```python
from build123d import *

# Parameters (mm, degrees)
RESSALTO_EXTRUS_O1_DEPTH = 30
ESBO_O2_R                = 5
CORTE_EXTRUS_O1_DEPTH    = 30
FILETE1_R                = 10


with BuildPart() as part:
    # Esboço1 → Ressalto-extrusão1 (new body)
    with BuildSketch(Plane.XY):
        with BuildLine():
            Line((-51.174680709, 2.345199545), (-29.908193511, 2.345199545))
            ThreePointArc((-29.908193511, 2.345199545), (0, 30), (29.908193511, 2.345199545))
            Line((29.908193511, 2.345199545), (51.174680709, 2.345199545))
            Line((51.174680709, 2.345199545), (78.983139003, 2.345199545))
            Line((78.983139003, 2.345199545), (78.983139003, 15))
            Line((78.983139003, 15), (48.983139003, 15))
            ThreePointArc((48.983139003, 15), (0, 51.228389654), (-48.983139003, 15))
            Line((-48.983139003, 15), (-78.983139003, 15))
            Line((-78.983139003, 15), (-78.983139003, 2.345199545))
            Line((-78.983139003, 2.345199545), (-51.174680709, 2.345199545))
        make_face()
    extrude(amount=RESSALTO_EXTRUS_O1_DEPTH)

    # Esboço2 → Corte-extrusão1 (cut)
    with BuildSketch(Plane(origin=(0, 15, 0), x_dir=(1, 0, 0), z_dir=(0, 1, 0))):
        with Locations(Location((-63.983139003, -15, 0), (0, 0, 180))):
            Circle(ESBO_O2_R)
        with Locations(Location((63.983139003, -15, 0), (0, 0, 180))):
            Circle(ESBO_O2_R)
    extrude(amount=-CORTE_EXTRUS_O1_DEPTH, mode=Mode.SUBTRACT)

    # Filete1
    filete1_edges = [part.edges().sort_by_distance(p)[0] for p in [
        (48.983139003, 15, 15),
        (-48.983139003, 15, 15),
    ]]
    fillet(filete1_edges, radius=FILETE1_R)


solid = part.part
```
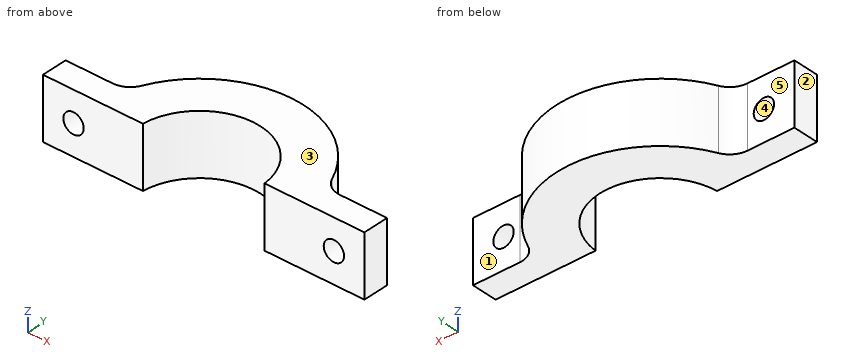
Verification items for the finished model (mm, model axes). Face numbers are marked on the shaded views. A direction names the side the tool comes from. Give positions to 0.01 mm unless a question says otherwise; leave off trailing zeros. Order: outer loops, then holes, each group sorted by start corner. A loop starts at its lowest first (then second) coordinate and runs counter-clockwise, first axis right, second up. Notation, with made-up numbers: (20, 84.5) -> (44, 84.5) arc R20 cw to (44, 99.5) -> close; hole circle Ø11 at (-29, 13). An arc over 180 degrees is marked (long way). One line per item, written item: value.
(1) Sectioned sample at B-B on z = 25.75. Record the cut outline in (x, y), then the cut area to 3 significant figures.
Final values:
outline: (-78.98, 2.35) -> (-29.91, 2.35) arc R30 cw to (29.91, 2.35) -> (78.98, 2.35) -> (78.98, 15) -> (55.89, 15) arc R10 cw to (46.76, 20.92) arc R51.23 ccw to (-46.76, 20.92) arc R10 cw to (-55.89, 15) -> (-78.98, 15) -> close
area: 3,350 mm^2
(2) Sectioned sample at D-D on x = -35. Record the cut outline in (y, z).
Final values:
outline: (2.35, 0) -> (37.41, 0) -> (37.41, 30) -> (2.35, 30) -> close
(3) Tool access check on the marked faces 1 and 2. Record the directions out of +Z, -Z, +X, -X, +Y, -Y that give a thin tool (end or side, any length) a straight path to the whole face; none if there is none.
Final values:
face 1: +Z, -Z, +X, +Y
face 2: +Z, -Z, -X, +Y, -Y
(4) Sectioned sample at C-C on x = 39.5. Record the cut outline in (y, z), then the cut area to 3 significant figures.
Final values:
outline: (2.35, 0) -> (32.62, 0) -> (32.62, 30) -> (2.35, 30) -> close
area: 908 mm^2
(5) Gauge pin test, flat ends, axial feed: pin 1 (8 mm diameter, centred on x = 63.98, z = 15, fed in from -Y); pin 2 (8 mm diameter, centred on x = 37, z = 25, fed in from +Y); pin 3 (3 mm diameter, centred on x = -29, z = 5, fed in from -Y); pin 4 (12 mm diameter, centred on y = 29.5, z = 24, fed in from -X). Record the tip position at first contact, or that the pin passes through.
Final values:
pin 1: through
pin 2: y = 39.18
pin 3: y = 2.35
pin 4: x = -45.52
(6) Scan lines: line 1 along X through (y, z) = (12.5, 12.5); line 2 along X through (y, z) = (26.5, 8); line 3 along X through (y, z) = (20, 19.75). Record each from-to range of solid material in increasing order. Write a range as [from, to].
Final values:
line 1: [-78.98, -68.31], [-59.65, -27.27], [27.27, 59.65], [68.31, 78.98]
line 2: [-43.84, -14.06], [14.06, 43.84]
line 3: [-47.23, -22.36], [22.36, 47.23]
(7) Sectioned sample at A-A on z = 15. Record the cut outline in (x, y).
Final values:
outline: (-78.98, 2.35) -> (-68.98, 2.35) -> (-68.98, 15) -> (-78.98, 15) -> close; (-58.98, 2.35) -> (-29.91, 2.35) arc R30 cw to (29.91, 2.35) -> (58.98, 2.35) -> (58.98, 15) -> (55.89, 15) arc R10 cw to (46.76, 20.92) arc R51.23 ccw to (-46.76, 20.92) arc R10 cw to (-55.89, 15) -> (-58.98, 15) -> close; (68.98, 2.35) -> (78.98, 2.35) -> (78.98, 15) -> (68.98, 15) -> close
(8) Draft check along Z on the marked faces 3, 4 and 5. Enter one of: pulls with the +Z half, pulls with the -Z half, needs draft (parallel to the pull), parting line crosses it, or undercut.
Final values:
face 3: pulls with the +Z half
face 4: undercut
face 5: needs draft
